Design review of the part built by this model. Coordinates are the model's own, in mm. A direction names the side the tool comes from. Give positions to 0.01 mm unless a question says otherwise; leave off trailing zeros. Order: outer loops, then holes, each group sorted by start corner. A loop starts at its lowest first (then second) coordinate and runs counter-clockwise, first axis right, second up. Notation, with made-up numbers: M -7.5,86.25 L 21.5,86.25 A26 cw 21.5,103.25 Z; hole C -32,-11.5 d3. An arc over 180 degrees is marked long. Put each result on its own line as item: value. Start each with the question number.
from build123d import *

# Parameters (mm, degrees)
F0_R      = 25
F1_DEPTH  = 1.5
F2_R      = 22.5
F3_DEPTH  = 18
F4_R      = 25
F5_DEPTH  = 1.5
F6_R      = 15
F7_DEPTH  = 5
F10_R     = 4
F11_DEPTH = 20


with BuildPart() as f1:
    # F0 (on Front) → F1 (new body)
    with BuildSketch(Plane.XZ):
        Circle(F0_R)
    extrude(amount=F1_DEPTH)

    # F2 (on face) → F3 (join)
    with BuildSketch(Plane.XZ.offset(1.5)):
        Circle(F2_R)
    extrude(amount=F3_DEPTH)

    # F4 (on face) → F5 (join)
    with BuildSketch(Plane.XZ.offset(19.5)):
        Circle(F4_R)
    extrude(amount=F5_DEPTH)

    # F6 (on face) → F7 (join)
    with BuildSketch(Plane.XZ.offset(21)):
        Circle(F6_R)
    extrude(amount=F7_DEPTH)

    # F8 (on Right) → F9 (revolve)
    with BuildSketch(Plane.YZ):
        Polygon((5, 0), (0, 0), (0, -8), (5, -2), align=None)
    revolve(axis=Axis((0, 10.197903, 0), (0, 1, 0)))

    # F10 (on face) → F11 (cut)
    with BuildSketch(Plane.XZ.offset(26)):
        Circle(F10_R)
    extrude(amount=-F11_DEPTH, mode=Mode.SUBTRACT)


solid = f1.part
1. The part is to be moulded in two halves that separate along Z. For faces 6 (the flat face through (-22.34, -19.5, 3.82)), 7 (the cylindrical face through (23.846, -20.24, 7.509)), 8 (the flat face through (0, -6, 0)), say which applies: +Z half, -Z half, draft (parallel to the pull), parting line (faces both ways), or undercut.
2. Machinability: for faces 1 (the cylindrical face through (10.382, -10.374, -19.961)), 2 (the cylindrical face through (23.846, -0.74, 7.509)), 3 (the flat face through (11, -21, -11)), 4 (the flat face through (-6, 0, 6)), 5 (the flat face through (0, 5, 0)), which of the approach directions +Z, -Z, +X, -X, +Y, -Y give a long, thin tool a straight path to every point of the face, cutting with its end or side? Answer none if there is none.
3. Insertion check: pin 1 (8 mm diameter, centred on y = -13.5, z = 15, fed in from -X); pin 2 (5 mm diameter, centred on x = -8, y = -8, fed in from -Z); pin 3 (15 mm diameter, centred on x = -5, z = -8.5, fed in from +Y). Each pin has a flat end and moves straight along its axis. Give the tip position at first contact, or say it passes through.
4. Consider section D-D on y = 2. Give the boundary of the cut face in (x, z), then the cut area to 3 significant figures.
5. Consider section B-B on z = 0. Give the boundary of the cut face in (x, y), then the cut area to 3 significant figures.
6. Consider section A-A on y = -8.5. Give the boundary of the cut face in (x, z).
7. To check wall thickness, follow probe 1 along Z at (x, y) = (0, -20.75); probe 2 along Z at (x, y) = (0, -10.25); probe 3 along Y at (x, z) = (-22, -4). State the ranges of each line that lie inside material, in increasing order.
8. Consider section C-C on x = 21.5. Give the boundary of the cut face in (y, z).
Returned:
1. face 6: draft
1. face 7: parting line
1. face 8: undercut
2. face 1: none
2. face 2: +Y, -Y
2. face 3: -Y
2. face 4: +Y
2. face 5: +Z, -Z, +X, -X, +Y
3. pin 1: stops at x = -19.63
3. pin 2: stops at z = -21.82
3. pin 3: stops at y = 4.7
4. outline: C 0,0 d11.2
4. area: 98.5 mm2
5. outline: M -25,-21 L -15,-21 L -15,-26 L -4,-26 L -4,-6 L 4,-6 L 4,-26 L 15,-26 L 15,-21 L 25,-21 L 25,-19.5 L 22.5,-19.5 L 22.5,-1.5 L 25,-1.5 L 25,0 L 8,0 L 2,5 L -2,5 L -8,0 L -25,0 L -25,-1.5 L -22.5,-1.5 L -22.5,-19.5 L -25,-19.5 Z
5. area: 1,000 mm2
6. outline: C 0,0 d45; hole C 0,0 d8
7. probe 1: z = -25 to -4, 4 to 25
7. probe 2: z = -22.5 to -4, 4 to 22.5
7. probe 3: y = -21 to 0
8. outline: M -21,-12.76 L -19.5,-12.76 L -19.5,-6.63 L -1.5,-6.63 L -1.5,-12.76 L 0,-12.76 L 0,12.76 L -1.5,12.76 L -1.5,6.63 L -19.5,6.63 L -19.5,12.76 L -21,12.76 Z
